Build history of the part. All positions in model axes, mm. A direction names the side the tool comes from. Give positions to 0.01 mm unless a question says otherwise; leave off trailing zeros. Write each loop counter-clockwise with the first axis right and the second up, starting at its lowest first coordinate (ties: lowest second). Pieces come first, ordered by that corner, then holes.
from build123d import *

# Parameters (mm, degrees)
SKETCH1_R           = 12.695
SKETCH1_W           = 14.99
SKETCH1_H           = 14.99
BOSS_EXTRUDE2_DEPTH = 20


with BuildPart() as part:
    # Sketch1 → Boss-Extrude2 (new body)
    with BuildSketch(Plane(origin=(0, 0, 0), x_dir=(1, 0, 0), z_dir=(0, 1, 0))):
        Circle(SKETCH1_R)
        Rectangle(SKETCH1_W, SKETCH1_H, mode=Mode.SUBTRACT)
    extrude(amount=BOSS_EXTRUDE2_DEPTH)


solid = part.part
(1) 3-axis set-ups, long thin cutter, end or side, ignore diameter. For faces 1 (the face through (0, 20, 8)), 2 (the face through (0, 10, -7.495)): which of +Z, -Z, +X, -X, +Y, -Y reach the whole face in a straight line?
(2) Drop a flat-ended pin along its axis: pin 1 (1.5 mm diameter, centred on y = 13.5, z = 8, fed in from +X). Give the stop position or say it passes through.
(3) Saw through at B-B, the plane x = 0. List the corners of the cut face in (y, z) (3 decimals).
(4) Mould opens along Z. For faces 3 (the face through (0, 10, 7.495)), 4 (the face through (0, 0, 8)), 5 (the face through (-10.074, 9.86, 7.725)), 6 (the face through (7.495, 10, 0)) say: +Z half, -Z half, draft (parallel to the pull), parting line (faces both ways), or undercut.
(5) Saw through at A-A, the plane z = 0. List the corners of the cut face in (x, y) (3 decimals).
(6) Saw through at C-C, the plane y = 7.25. List the corners of the cut face in (x, z) (3 decimals).
(7) Saw through at D-D, the plane z = -8.75. List the corners of the cut face in (x, y), plus the area to 3 significant figures.
(8) Probe line 1 (Z direction, x = 0, y = 18.5) (3 decimals); line 2 (Z direction, x = -4.25, y = 5.5) (3 decimals); line 3 (X direction, y = 8.75, z = 4.75) (3 decimals). List the from-to ranges inside material, lowest first.
Computed values:
1. face 1: +Z, -Z, +X, -X, +Y
1. face 2: +Y, -Y
2. pin 1: stops at x = 10.42
3. outline: (0, -12.695) - (20, -12.695) - (20, -7.495) - (0, -7.495) - close; (0, 7.495) - (20, 7.495) - (20, 12.695) - (0, 12.695) - close
4. face 3: undercut
4. face 4: draft
4. face 5: parting line
4. face 6: undercut
5. outline: (-12.695, 0) - (-7.495, 0) - (-7.495, 20) - (-12.695, 20) - close; (7.495, 0) - (12.695, 0) - (12.695, 20) - (7.495, 20) - close
6. outline: circle Ø25.39 at (0, 0); hole (-7.495, -7.495) - (7.495, -7.495) - (7.495, 7.495) - (-7.495, 7.495) - close
7. outline: (-9.2, 0) - (9.2, 0) - (9.2, 20) - (-9.2, 20) - close
7. area: 368 mm2
8. line 1: z = -12.695 to -7.495, 7.495 to 12.695
8. line 2: z = -11.962 to -7.495, 7.495 to 11.962
8. line 3: x = -11.773 to -7.495, 7.495 to 11.773
